For this review, take the finished solid that the model builds, in its own axes (mm). A direction names the side the tool comes from. Coordinates: 2 decimals unless noted, no trailing zeros. Write each loop counter-clockwise with the first axis right and the second up, starting at its lowest first coordinate (ties: lowest second). Pieces come first, ordered by that corner, then holes. Notation, with made-up numbers: (17, 24) - (62, 24) arc R30 cw to (62, 57) - close; hole circle Ø7 at (37.25, 65). An arc over 180 degrees is marked (long way). Write each question's results on one line, items separated by ' | '.
from build123d import *

# Parameters (mm, degrees)
FILLET1_R     = 2
SCALE_1_SCALE = 0.6


with BuildPart() as part:
    # Sketch1 → Revolve1 (revolve)
    with BuildSketch(Plane.XY, mode=Mode.PRIVATE) as revolve1_sk:
        with BuildLine():
            Line((0, -42), (0, 37.091148677))
            ThreePointArc((0, 37.091148677), (2.291287847, 36.02764035), (2.958039892, 33.591148677))
            ThreePointArc((2.958039892, 33.591148677), (8.355680086, 28.435189692), (8.005599308, 20.978925468))
            ThreePointArc((8.005599308, 20.978925468), (6.920726173, 17.042188603), (7.5, 13))
            Line((7.5, 13), (10, 13))
            Line((10, 13), (10, 10))
            Line((10, 10), (8, 10))
            Line((8, 10), (8, 8))
            ThreePointArc((8, 8), (6.5, 6.5), (8, 5))
            Line((8, 5), (8, 3))
            Line((8, 3), (12.5, 3))
            Line((12.5, 3), (12.5, 0))
            Line((12.5, 0), (7.5, 0))
            ThreePointArc((7.5, 0), (10.655312326, -19.545502593), (20, -37))
            Line((20, -37), (20, -42))
            Line((20, -42), (0, -42))
        make_face()
    revolve(revolve1_sk.sketch.rotate(Axis((0, 46.430278851, 0), (0, -1, 0)), 90), axis=Axis((0, 46.430278851, 0), (0, -1, 0)))

    # Fillet1
    fillet1_edges = [part.edges().sort_by_distance(p)[0] for p in [
        (0, 0, -7.5),
    ]]
    fillet(fillet1_edges, radius=FILLET1_R)


with BuildPart() as part_1:
    # 缩放比例1: scaled about (0, 0, 0)
    add(part.part.scale(SCALE_1_SCALE))


solid = part_1.part
Q1. Wall thickness on line 1 along Y through (x, z) = (-5.5, -4); line 2 along Y through (x, z) = (-3.25, -6.5); line 3 along Y through (x, z) = (-3.5, 1.5): over which ranges is each line inside the solid? List them lowest first. Write a range as from..to.
Results found:
line 1: -25.2..-12.87, 0..1.8 | line 2: -25.2..-14.05, 0..1.8 | line 3: -25.2..18.88
Q2. For faces 4 (the face through (-3.604, -23.721, 11.446)), 5 (the face through (-4.05, 2.39, 2.58)), 6 (the face through (-1.802, 6.887, 5.723)), list the 3-axis set-ups (+Z, -Z, +X, -X, +Y, -Y) from which the entire face can be reached by the end or side of a thin tool; tool diameter is ignored.
Results found:
face 4: +Y, -Y | face 5: none | face 6: +Y
Q3. Take a section at B-B on y = -19. State the section outline as (x, z) points, plus the area to 3 significant figures.
Results found:
outline: circle Ø19.59 at (0, 0) | area: 301 mm2
Q4. For pin 1 (9.5 mm diameter, centred on x = 0.5, z = 2.5, fed in from +Y); pin 2 (12 mm diameter, centred on x = -3, z = -8.5, fed in from +Y); pin 3 (1 mm diameter, centred on x = 5.5, z = -5.5, fed in from +Y); pin 4 (2 mm diameter, centred on x = 0.5, z = -6.5, fed in from +Y), all flat-tipped, find the tip position at first contact; note any pin that passes through.
Results found:
pin 1: y = 22.25 | pin 2: y = 19.54 | pin 3: y = 1.8 | pin 4: y = 7.8
Q5. Take a section at A-A on y = 15. State the section outline as (x, z) points.
Results found:
outline: circle Ø10.8 at (0, 0)
Q6. Mouldability with a two-part tool opening along Y and no side actions: class faces 1 (the face through (0, -25.2, 0)), 2 (the face through (-4, 6, -3)), 3 (the face through (-6.324, 0.887, 4.032)) as pulls with the +Y half, pulls with the -Y half, needs draft (parallel to the pull), parting line crosses it, or undercut.
Results found:
face 1: pulls with the -Y half | face 2: undercut | face 3: needs draft
